Geometry: see drawing. Coordinates: mm, zero at the bounding-box minimum. Coordinates: 2 decimals unless noted, no trailing zeros. Order: outer loops, then holes, each group sorted by start corner. A loop starts at its lowest first (then second) coordinate and runs counter-clockwise, first axis right, second up. Notation, with made-up numbers: M 17,-24 L 43,-24 A30 ccw 43,0 Z; hole C 17,-14 d6. An arc over 180 degrees is marked long. One line per item, written item: value.
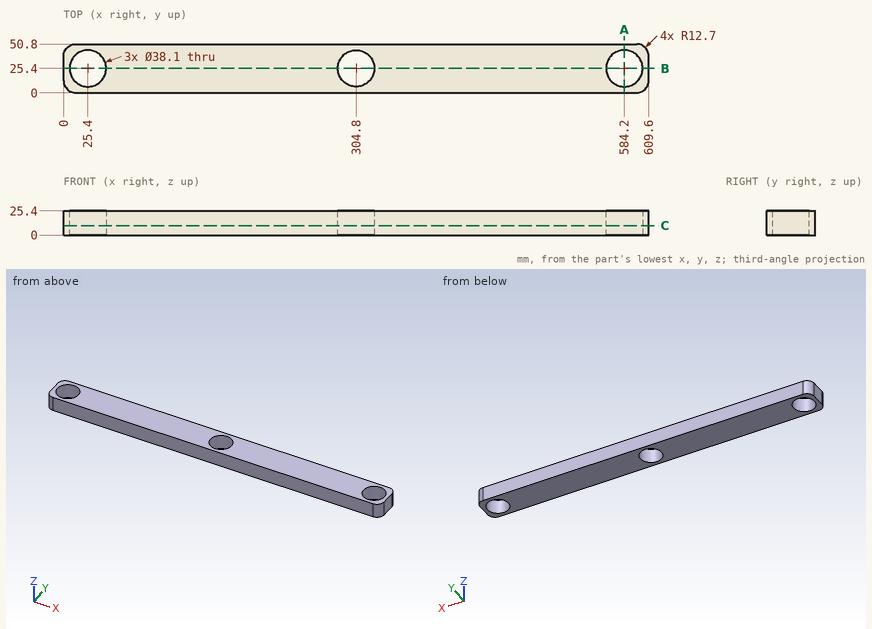
(1) Cut plane A-A on x = 584.2. Output: boundary loops of the cut face in (y, z).
Data:
outline: M 0,0 L 6.35,0 L 6.35,25.4 L 0,25.4 Z; M 44.45,0 L 50.8,0 L 50.8,25.4 L 44.45,25.4 Z
(2) Cut plane C-C on z = 10. Output: boundary loops of the cut face in (x, y), plus the area to 3 significant figures.
Data:
outline: M 0,12.7 A12.7 ccw 12.7,0 L 596.9,0 A12.7 ccw 609.6,12.7 L 609.6,38.1 A12.7 ccw 596.9,50.8 L 12.7,50.8 A12.7 ccw 0,38.1 Z; hole C 25.4,25.4 d38.1; hole C 304.8,25.4 d38.1; hole C 584.2,25.4 d38.1
area: 27,400 mm2
(3) First-contact query: pin 1 (2 mm diameter, centred on y = 8, z = 5, fed in from +X). Flat tip, straight axial feed; report the tip coordinate or a pass-through.
Data:
pin 1: stops at x = 609.05
(4) Cut plane B-B on y = 25.4. Output: boundary loops of the cut face in (x, z).
Data:
outline: M 0,0 L 6.35,0 L 6.35,25.4 L 0,25.4 Z; M 44.45,0 L 285.75,0 L 285.75,25.4 L 44.45,25.4 Z; M 323.85,0 L 565.15,0 L 565.15,25.4 L 323.85,25.4 Z; M 603.25,0 L 609.6,0 L 609.6,25.4 L 603.25,25.4 Z
(5) Ray query, line 1 (X direction, y = 28, z = 7.75); line 2 (X direction, y = 30, z = 23.5); line 3 (Y direction, x = 583.5, z = 18.5). Return the intervals inside material, ascending. Write a range as from..to.
Data:
line 1: x = 0..6.53, 44.27..285.93, 323.67..565.33, 603.07..609.6
line 2: x = 0..6.91, 43.89..286.31, 323.29..565.71, 602.69..609.6
line 3: y = 0..6.36, 44.44..50.8
